For this review, take the finished solid that the model builds, in its own axes (mm). Round coordinates to 2 decimals unless told otherwise and drop trailing zeros. Order: outer loops, then holes, each group sorted by start corner. A loop starts at its lowest first (then second) coordinate and runs counter-clockwise, first axis right, second up. Notation, with made-up numbers: (16.5, -25) - (31.5, -25) arc R19 cw to (31.5, 9) - close; hole circle Ø9 at (-9, 82). An arc over 180 degrees is marked (long way). Write each question's results on one line, items separated by ' | '. Start each with the question number.
(1) For L1, parallel to Y at x = -186.5, z = 10; L2, parallel to X at y = 2, z = 8.5; L3, parallel to Z at x = 181, y = 8.25, list the stretches that pass through material, from the lowest coordinate up. Write a range as from..to.
(2) Insertion check: pin 1 Ø3 at (x, z) = (222, 6.5) entering from +Y; pin 2 Ø7.5 at (x, z) = (221.5, 5.5) entering from -Y; pin 3 Ø2.5 at (y, z) = (1, 9) entering from -X. Each pin has a flat end and moves straight along its axis. Give the tip position at first contact, or say it passes through.
(3) Take a section at A-A, the plane z = 8. Give the boundary of the cut face in (x, y) (3 decimals), plus the area to 3 significant figures.
(4) Take a section at B-B, the plane x = -60.5. Give the boundary of the cut face in (y, z), plus the area to 3 significant figures.
```python
from build123d import *

# Parameters (mm, degrees)
F0_W     = 19.05
F0_H     = 12.7
F1_DEPTH = 225.425
F2_W     = 3.96875
F2_H     = 7.14375
F3_DEPTH = 450.85
F4_W     = 9.525
F4_H     = 2.38125
F5_DEPTH = 12.7


# Not quite as in the source:
# - a pattern or mirror of a feature is missing from the dataset's text; its kind, count and spacing are read off the source's solid


with BuildPart() as f1:
    # F0 (on Right) → F1 (new body, symmetric)
    with BuildSketch(Plane.YZ):
        with Locations((9.525, 6.35)):
            Rectangle(F0_W, F0_H)
    extrude(amount=F1_DEPTH, both=True)

    # F2 (on face) → F3 (cut, through all)
    with BuildSketch(Plane.YZ.offset(225.425)):
        with Locations((9.525, 9.128125)):
            Rectangle(F2_W, F2_H)
    extrude(amount=-F3_DEPTH, mode=Mode.SUBTRACT)

    # F4 (on face) → F5 (cut, through all)
    with BuildSketch(Plane.XY.offset(12.7)):
        with Locations((220.6625, 17.859375)):
            Rectangle(F4_W, F4_H)
        with Locations((220.6625, 1.190625)):
            Rectangle(F4_W, F4_H)
    f5 = extrude(amount=-F5_DEPTH, mode=Mode.SUBTRACT)

    # F5_copies: F5 across plane
    add(f5.mirror(Plane(origin=(0, 0, 0), x_dir=(0, 0, -1), z_dir=(-1, 0, 0))), mode=Mode.SUBTRACT)


solid = f1.part
```
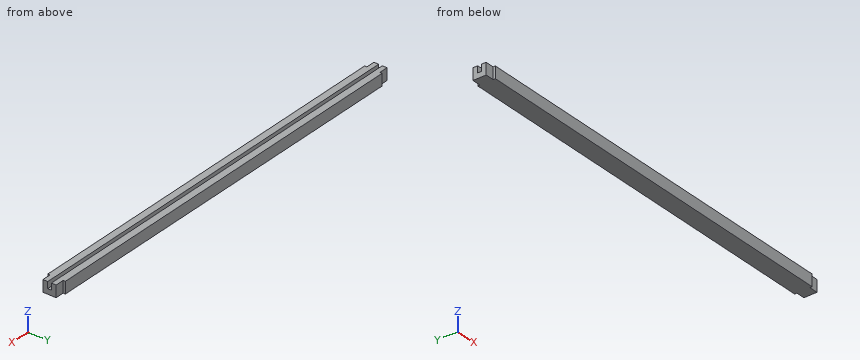
Results below:
1) L1: y = 0..7.54, 11.51..19.05 | L2: x = -215.9..215.9 | L3: z = 0..5.56
2) pin 1: stops at y = 16.67 | pin 2: stops at y = 2.38 | pin 3: stops at x = -215.9
3) outline: (-225.425, 2.381) - (-215.9, 2.381) - (-215.9, 0) - (215.9, 0) - (215.9, 2.381) - (225.425, 2.381) - (225.425, 7.541) - (-225.425, 7.541) - close; (-225.425, 11.509) - (225.425, 11.509) - (225.425, 16.669) - (215.9, 16.669) - (215.9, 19.05) - (-215.9, 19.05) - (-215.9, 16.669) - (-225.425, 16.669) - close | area: 6,710 mm^2
4) outline: (0, 0) - (19.05, 0) - (19.05, 12.7) - (11.51, 12.7) - (11.51, 5.56) - (7.54, 5.56) - (7.54, 12.7) - (0, 12.7) - close | area: 214 mm^2
